Geometry: final body of the model. Coordinates: model frame, mm. A direction names the side the tool comes from. Coordinates: 2 decimals unless noted, no trailing zeros. Loops run counter-clockwise (first coordinate to the right, second up) from the corner with the lowest first, then second, coordinate; pieces in that order, holes last. Notation, with made-up numbers: M -13.75,-27.5 L 1.25,-27.5 A8 ccw 1.25,-15.5 Z; hole C -37.5,-12 d8. An arc over 180 degrees is marked long. Write each question's results on one line, items separated by ' | '. Start each with the question number.
from build123d import *

# Parameters (mm, degrees)
SKETCH1_R           = 30.25
SKETCH1_R_2         = 25.25
EXTRUDE_THIN1_DEPTH = 3
SKETCH2_R           = 1.65
CUT_EXTRUDE3_DEPTH  = 10
BOSS_EXTRUDE1_DEPTH = 3


with BuildPart() as part:
    # Sketch1 → Extrude-Thin1 (new body)
    with BuildSketch(Plane(origin=(0, 0, 0), x_dir=(1, 0, 0), z_dir=(0, 1, 0))):
        Circle(SKETCH1_R)
        Circle(SKETCH1_R_2, mode=Mode.SUBTRACT)
    extrude(amount=-EXTRUDE_THIN1_DEPTH)

    # Sketch2 → Cut-Extrude3 (cut)
    with BuildSketch(Plane(origin=(0, 0, 0), x_dir=(1, 0, 0), z_dir=(0, 1, 0))):
        with Locations((0, 27.5)):
            Circle(SKETCH2_R)
        with Locations((23.815698604, -13.75)):
            Circle(SKETCH2_R)
        with Locations((-23.815698604, -13.75)):
            Circle(SKETCH2_R)
    extrude(amount=-CUT_EXTRUDE3_DEPTH, mode=Mode.SUBTRACT)

    # Sketch5 → Boss-Extrude1 (add)
    with BuildSketch(Plane.XZ.offset(3)):
        with BuildLine():
            Line((0, 58.25), (0, 30.25))
            ThreePointArc((0, 30.25), (2.899334014, 30.110735001), (5.77197211, 29.694222299))
            Line((5.77197211, 29.694222299), (11.114623981, 57.179783436))
            ThreePointArc((11.114623981, 57.179783436), (5.583015084, 57.981828555), (0, 58.25))
        make_face()
        with BuildLine():
            Line((29.125, 50.44597977), (15.125, 26.197268464))
            ThreePointArc((15.125, 26.197268464), (17.56626441, 24.62699443), (19.845785627, 22.829964802))
            Line((19.845785627, 22.829964802), (38.215438439, 43.961833048))
            ThreePointArc((38.215438439, 43.961833048), (33.82594717, 47.422228944), (29.125, 50.44597977))
        make_face()
        with BuildLine():
            Line((50.44597977, 29.125), (26.197268464, 15.125))
            ThreePointArc((26.197268464, 15.125), (27.526328444, 12.54447059), (28.601936912, 9.848436672))
            Line((28.601936912, 9.848436672), (55.076457029, 18.964344997))
            ThreePointArc((55.076457029, 18.964344997), (53.005244029, 24.155881385), (50.44597977, 29.125))
        make_face()
        with BuildLine():
            Line((58.25, 0), (30.25, 0))
            ThreePointArc((30.25, 0), (30.110735001, -2.899334014), (29.694222299, -5.77197211))
            Line((29.694222299, -5.77197211), (57.179783436, -11.114623981))
            ThreePointArc((57.179783436, -11.114623981), (57.981828555, -5.583015084), (58.25, 0))
        make_face()
        with BuildLine():
            Line((50.44597977, -29.125), (26.197268464, -15.125))
            ThreePointArc((26.197268464, -15.125), (24.62699443, -17.56626441), (22.829964802, -19.845785627))
            Line((22.829964802, -19.845785627), (43.961833048, -38.215438439))
            ThreePointArc((43.961833048, -38.215438439), (47.422228944, -33.82594717), (50.44597977, -29.125))
        make_face()
        with BuildLine():
            Line((29.125, -50.44597977), (15.125, -26.197268464))
            ThreePointArc((15.125, -26.197268464), (12.54447059, -27.526328444), (9.848436672, -28.601936912))
            Line((9.848436672, -28.601936912), (18.964344997, -55.076457029))
            ThreePointArc((18.964344997, -55.076457029), (24.155881385, -53.005244029), (29.125, -50.44597977))
        make_face()
        with BuildLine():
            Line((0, -58.25), (0, -30.25))
            ThreePointArc((0, -30.25), (-2.899334014, -30.110735001), (-5.77197211, -29.694222299))
            Line((-5.77197211, -29.694222299), (-11.114623981, -57.179783436))
            ThreePointArc((-11.114623981, -57.179783436), (-5.583015084, -57.981828555), (0, -58.25))
        make_face()
        with BuildLine():
            Line((-29.125, -50.44597977), (-15.125, -26.197268464))
            ThreePointArc((-15.125, -26.197268464), (-17.56626441, -24.62699443), (-19.845785627, -22.829964802))
            Line((-19.845785627, -22.829964802), (-38.215438439, -43.961833048))
            ThreePointArc((-38.215438439, -43.961833048), (-33.82594717, -47.422228944), (-29.125, -50.44597977))
        make_face()
        with BuildLine():
            Line((-50.44597977, -29.125), (-26.197268464, -15.125))
            ThreePointArc((-26.197268464, -15.125), (-27.526328444, -12.54447059), (-28.601936912, -9.848436672))
            Line((-28.601936912, -9.848436672), (-55.076457029, -18.964344997))
            ThreePointArc((-55.076457029, -18.964344997), (-53.005244029, -24.155881385), (-50.44597977, -29.125))
        make_face()
        with BuildLine():
            Line((-58.25, 0), (-30.25, 0))
            ThreePointArc((-30.25, 0), (-30.110735001, 2.899334014), (-29.694222299, 5.77197211))
            Line((-29.694222299, 5.77197211), (-57.179783436, 11.114623981))
            ThreePointArc((-57.179783436, 11.114623981), (-57.981828555, 5.583015084), (-58.25, 0))
        make_face()
        with BuildLine():
            Line((-50.44597977, 29.125), (-26.197268464, 15.125))
            ThreePointArc((-26.197268464, 15.125), (-24.62699443, 17.56626441), (-22.829964802, 19.845785627))
            Line((-22.829964802, 19.845785627), (-43.961833048, 38.215438439))
            ThreePointArc((-43.961833048, 38.215438439), (-47.422228944, 33.82594717), (-50.44597977, 29.125))
        make_face()
        with BuildLine():
            Line((-29.125, 50.44597977), (-15.125, 26.197268464))
            ThreePointArc((-15.125, 26.197268464), (-12.54447059, 27.526328444), (-9.848436672, 28.601936912))
            Line((-9.848436672, 28.601936912), (-18.964344997, 55.076457029))
            ThreePointArc((-18.964344997, 55.076457029), (-24.155881385, 53.005244029), (-29.125, 50.44597977))
        make_face()
    extrude(amount=-BOSS_EXTRUDE1_DEPTH)


solid = part.part
Item 1: Section B-B, the plane x = 17.5. Return loops of the section in (y, z).
Item 2: Contact query for flat-ended pins moving along their axis: P1, Ø1, axis at y = -1.5, z = 35.5, coming from the +X side; P2, Ø0.9, axis at x = -42.5, y = -1, coming from the -Z side; P3, Ø1.5, axis at y = -1.5, z = 39.5, coming from the -X side. Output: stop coordinate, or through.
Item 3: Ray query, L1, parallel to Z at x = 45, y = -1.65; L2, parallel to X at y = -0.95, z = 30.5; L3, parallel to Z at x = 20, y = -2.5. Return the intervals inside material, ascending. Write a range as [from, to].
Item 4: Section A-A, the plane z = -41. Return loops of the section in (x, y).
Item 5: Section D-D, the plane y = -1.25. Count the separate pieces of the cut face and the enclosed holes in it, plus the area to 3 significant figures.
Item 6: Pull-direction query (Z, two-part tool) for faces 6 (the cylindrical face through (47.377, -1.521, -33.89)), 7 (the cylindrical face through (-28.36, -1.48, 10.53)), 8 (the cylindrical face through (-57.974, -1.521, 5.661)); classes: released by +Z, released by -Z, zero draft, split by the parting line, or undercut.
Item 7: Set-up query: faces 1 (the cylindrical face through (-10.53, -1.48, -28.36)), 2 (the flat face through (-22.22, -1.52, -38.49)), 3 (the cylindrical face through (-29.823, -1.479, -5.062)), 4 (the cylindrical face through (-5.062, -1.479, 29.823)), 5 (the flat face through (41.65, -1.52, 14.34)). Return all of +Z, -Z, +X, -X, +Y, -Y with unobstructed straight access to the full face (end or side cutting, diameter ignored); none if empty.
Item 8: Section C-C, the plane z = 13.75. Return loops of the section in (x, y), plus the area to 3 significant figures.
Solutions:
1) outline: M -3,-50.82 L 0,-50.82 L 0,-30.31 L -3,-30.31 Z; M -3,-24.67 L 0,-24.67 L 0,-18.2 L -3,-18.2 Z; M -3,18.2 L 0,18.2 L 0,30.31 L -3,30.31 Z
2) P1: stops at x = 31.29 | P2: stops at z = -24.8 | P3: stops at x = -23.24
3) L1: z = [-36.99, -25.98], [-8.75, 0], [15.49, 25.98] | L2: x = [-49.63, -35.09], [-17.61, -10.5], [0, 5.93], [17.61, 26.51] | L3: z = [-54.71, -34.64], [-22.69, -15.41], [15.41, 22.69], [23.01, 34.64]
4) outline: M -35.64,-3 L -23.67,-3 L -23.67,0 L -35.64,0 Z; M -7.97,-3 L 0,-3 L 0,0 L -7.97,0 Z; M 14.12,-3 L 23.67,-3 L 23.67,0 L 14.12,0 Z
5) separate pieces: 1 | enclosed holes: 4 | area: 3,700 mm²
6) face 6: released by -Z | face 7: undercut | face 8: released by +Z
7) face 1: +Y, -Y | face 2: -Z, +Y, -Y | face 3: -X, +Y, -Y | face 4: +Z, +Y, -Y | face 5: +X, +Y, -Y
8) outline: M -26.94,-3 L -25.47,-3 L -25.47,0 L -26.94,0 Z; M -22.17,-3 L -21.18,-3 L -21.18,0 L -22.17,0 Z; M 21.18,-3 L 22.17,-3 L 22.17,0 L 21.18,0 Z; M 25.47,-3 L 39.93,-3 L 39.93,0 L 25.47,0 Z | area: 53.8 mm²
